Verification items for the finished model (mm, model axes). A direction names the side the tool comes from. Coordinates: 2 decimals unless noted, no trailing zeros. Write each loop counter-clockwise with the first axis right and the second up, starting at its lowest first coordinate (ties: lowest second). Pieces come first, ordered by that corner, then holes. Notation, with made-up numbers: (48.5, -38) -> (79.5, -38) arc R33 ccw to (79.5, -6) -> close; hole circle Ø10 at (-16.75, -32). An arc over 180 degrees is marked (long way). Write item = value, one per line. Start each with the question number.
(1) Section check C-C (z = -0.5). Record the cut outline in (x, y).
(2) Set-up check for faces 5 (the face through (11.5, 6.5, -9.5)), 6 (the face through (14, 3, -7)), 7 (the face through (-13.5, -1, -15)), 8 (the face through (0, 7.5, 13)), 9 (the face through (13.5, -1, -16)): record each of +Z, -Z, +X, -X, +Y, -Y from which the full face is reachable in a straight line by a thin tool's end or side.
(3) Gauge pin test, flat ends, axial feed: pin 1 Ø1 at (y, z) = (-0.5, -16.5) entering from -X; pin 2 Ø2 at (y, z) = (-1, -4.5) entering from +X; pin 3 Ø2 at (x, z) = (-11, -6.5) entering from +Y. Record the tip position at first contact, or that the pin passes through.
(4) Mould release check, pull along Z, two halves, no side actions. Record for faces 1 (the face through (5.81, -1.01, -5.87)), 2 (the face through (-14, 3, -12)), 3 (the face through (0, 5.5, 13)), 4 (the face through (0, 4, 14.5)): released by +Z, released by -Z, zero draft, split by the parting line, or undercut.
(5) Section check D-D (x = -10). Record the cut outline in (y, z), plus the area to 3 significant figures.
(6) Section check B-B (x = 4.5). Record the cut outline in (y, z).
(7) Section check A-A (y = 6). Record the cut outline in (x, z), plus the area to 3 significant figures.
(8) Material ranges on probe 1 along Y at (x, z) = (13, -10); probe 2 along Y at (x, z) = (-12.75, -12.5); probe 3 along Z at (x, y) = (-0.25, 1), recorded low to high. Write a range as [from, to].
```python
from build123d import *

# Parameters (mm, degrees)
F1_DEPTH  = 2
F4_DEPTH  = 1
F6_DEPTH  = 2
F9_DEPTH  = 1
F12_DEPTH = 1
F13_W     = 2
F13_H     = 2
F14_ANGLE = 180
F15_W     = 2
F15_H     = 2
F16_ANGLE = 180
F17_W     = 2
F17_H     = 2
F18_ANGLE = 180
F19_R     = 5.5
F20_DEPTH = 5


# Not quite as in the source:
# - a feature names something its author has since deleted; it is built from what else it names


with BuildPart() as f1:
    # F0 (on Front) → F1 (new body)
    with BuildSketch(Plane.XZ):
        with BuildLine():
            ThreePointArc((-13.5, 0), (0, -13.5), (13.5, 0))
            ThreePointArc((13.5, 0), (0, 13.5), (-13.5, 0))
        make_face()
        with BuildLine():
            Line((13.5, -19), (13.5, 0))
            ThreePointArc((13.5, 0), (0, -13.5), (-13.5, 0))
            Line((-13.5, 0), (-13.5, -19))
            Line((-13.5, -19), (13.5, -19))
        make_face()
    extrude(amount=F1_DEPTH)

    # F3 (on offset) → F4 (join)
    with BuildSketch(Plane.XY.offset(13.5)):
        with BuildLine():
            Line((-2.5, 7.5), (-2.5, -2))
            Line((-2.5, -2), (2.5, -2))
            Line((2.5, -2), (2.5, 7.5))
            ThreePointArc((2.5, 7.5), (1.767766953, 9.267766953), (0, 10))
            ThreePointArc((0, 10), (-1.767766953, 9.267766953), (-2.5, 7.5))
        make_face()
    extrude(amount=F4_DEPTH)

    # F5 (on face) → F6 (join)
    with BuildSketch(Plane.XZ.offset(2)):
        with BuildLine():
            Line((-2.5, 13.5), (-2.5, 13.2664991614))
            ThreePointArc((-2.5, 13.2664991614), (-1.2554404249, 13.4414980318), (0, 13.5))
            Line((0, 13.5), (-2.5, 13.5))
        make_face()
        with BuildLine():
            ThreePointArc((0, 13.5), (1.2554404249, 13.4414980318), (2.5, 13.2664991614))
            Line((2.5, 13.2664991614), (2.5, 13.5))
            Line((2.5, 13.5), (0, 13.5))
        make_face()
    extrude(amount=-F6_DEPTH)

    # F8 (on offset) → F9 (join)
    with BuildSketch(Plane.YZ.offset(13.5)):
        with BuildLine():
            Line((7.5, -7), (-2, -7))
            Line((-2, -7), (-2, -12))
            Line((-2, -12), (7.5, -12))
            ThreePointArc((7.5, -12), (9.267766953, -11.267766953), (10, -9.5))
            ThreePointArc((10, -9.5), (9.267766953, -7.732233047), (7.5, -7))
        make_face()
    extrude(amount=F9_DEPTH)

    # F11 (on offset) → F12 (join)
    with BuildSketch(Plane.YZ.offset(-13.5)):
        with BuildLine():
            Line((7.5, -7), (-2, -7))
            Line((-2, -7), (-2, -12))
            Line((-2, -12), (7.5, -12))
            ThreePointArc((7.5, -12), (9.267766953, -11.267766953), (10, -9.5))
            ThreePointArc((10, -9.5), (9.267766953, -7.732233047), (7.5, -7))
        make_face()
    extrude(amount=-F12_DEPTH)

    # F13 (on face) → F14 (revolve)
    with BuildSketch(Plane(origin=(0, 0, 13.5), x_dir=(1, 0, 0), z_dir=(0, 0, -1))):
        with Locations((-1, -6.5)):
            Rectangle(F13_W, F13_H)
    revolve(axis=Axis((0, 6.5, 13.5), (0, -1, 0)), revolution_arc=F14_ANGLE)

    # F15 (on face) → F16 (revolve)
    with BuildSketch(Plane(origin=(13.5, 0, 0), x_dir=(0, -1, 0), z_dir=(-1, 0, 0))):
        with Locations((-6.5, -8.5)):
            Rectangle(F15_W, F15_H)
    revolve(axis=Axis((13.5, 6.5, -9.5), (0, -1, 0)), revolution_arc=F16_ANGLE)

    # F17 (on face) → F18 (revolve)
    with BuildSketch(Plane.YZ.offset(-13.5)):
        with Locations((6.5, -8.5)):
            Rectangle(F17_W, F17_H)
    revolve(axis=Axis((-13.5, 6.5, -9.5), (0, 1, 0)), revolution_arc=F18_ANGLE)

    # F19 (on face) → F20 (cut)
    with BuildSketch(Plane.XZ.offset(2)):
        with Locations((-7.0192593016, -0.5)):
            Circle(F19_R)
        with Locations((7, -0.5)):
            Circle(F19_R)
    extrude(amount=-F20_DEPTH, mode=Mode.SUBTRACT)


solid = f1.part
```
Response:
q1.outline = (-13.5, -2) -> (-12.52, -2) -> (-12.52, 0) -> (-13.5, 0) -> close; (-1.52, -2) -> (1.5, -2) -> (1.5, 0) -> (-1.52, 0) -> close; (12.5, -2) -> (13.5, -2) -> (13.5, 0) -> (12.5, 0) -> close
q2.face_5 = +Y
q2.face_6 = +Z, +X, +Y, -Y
q2.face_7 = -Z, -X, +Y, -Y
q2.face_8 = -Z, +X, -X, +Y
q2.face_9 = -Z, +X, +Y, -Y
q3.pin_1 = -13.5
q3.pin_2 = 13.5
q3.pin_3 = 0
q4.face_1 = undercut
q4.face_2 = released by -Z
q4.face_3 = zero draft
q4.face_4 = released by +Z
q5.outline = (-2, -19) -> (0, -19) -> (0, -5.12) -> (-2, -5.12) -> close; (-2, 4.12) -> (0, 4.12) -> (0, 9.07) -> (-2, 9.07) -> close
q5.area = 37.6 mm2
q6.outline = (-2, -19) -> (0, -19) -> (0, -5.4) -> (-2, -5.4) -> close; (-2, 4.4) -> (0, 4.4) -> (0, 12.73) -> (-2, 12.73) -> close
q7.outline = (-14.5, -12) -> (-13.5, -12) -> (-13.5, -11.5) arc R2 ccw to (-13.5, -7.5) -> (-13.5, -7) -> (-14.5, -7) -> close; (-2.5, 13.5) -> (-2, 13.5) arc R2 ccw to (2, 13.5) -> (2.5, 13.5) -> (2.5, 14.5) -> (-2.5, 14.5) -> close; (13.5, -12) -> (14.5, -12) -> (14.5, -7) -> (13.5, -7) -> (13.5, -7.5) arc R2 ccw to (13.5, -11.5) -> close
q7.area = 33.8 mm2
q8.probe_1 = [-2, 0], [5.5, 7.5]
q8.probe_2 = [-2, 0]
q8.probe_3 = [13.5, 14.5]
